```python
from build123d import *

# Parameters (mm, degrees)
SKETCH1_R           = 12.7
BOSS_EXTRUDE1_DEPTH = 622.3
SKETCH2_OUTSIDE_W   = 152.068
SKETCH2_OUTSIDE_H   = 152.068
SKETCH2_OUTSIDE_R   = 6.361935525
CUT_EXTRUDE1_DEPTH  = 38.1
SKETCH5_OUTSIDE_W   = 152.068
SKETCH5_OUTSIDE_H   = 152.068
SKETCH5_OUTSIDE_R   = 6.377907631
CUT_EXTRUDE4_DEPTH  = 38.1


with BuildPart() as part:
    # Sketch1 → Boss-Extrude1 (new body)
    with BuildSketch(Plane.XY):
        Circle(SKETCH1_R)
    extrude(amount=BOSS_EXTRUDE1_DEPTH)

    # Sketch2 outside → Cut-Extrude1 (cut)
    with BuildSketch(Plane.XY):
        Rectangle(SKETCH2_OUTSIDE_W, SKETCH2_OUTSIDE_H)
        with Locations(Location((0, 0, 0), (0, 0, 180))):
            Circle(SKETCH2_OUTSIDE_R, mode=Mode.SUBTRACT)
    extrude(amount=CUT_EXTRUDE1_DEPTH, mode=Mode.SUBTRACT)

    # Sketch5 outside → Cut-Extrude4 (cut)
    with BuildSketch(Plane.XY.offset(622.3)):
        Rectangle(SKETCH5_OUTSIDE_W, SKETCH5_OUTSIDE_H)
        Circle(SKETCH5_OUTSIDE_R, mode=Mode.SUBTRACT)
    extrude(amount=-CUT_EXTRUDE4_DEPTH, mode=Mode.SUBTRACT)


solid = part.part
```
Can you work these out from the model? Positions are in its coordinate system, mm. A direction names the side the tool comes from. Coordinates: 2 decimals unless noted, no trailing zeros. Order: outer loops, then holes, each group sorted by start corner. A loop starts at its lowest first (then second) coordinate and runs counter-clockwise, first axis right, second up. Notation, with made-up numbers: (16.25, 76) - (47.25, 76) arc R25 cw to (47.25, 102) - close; hole circle Ø5 at (26, -25). An arc over 180 degrees is marked (long way). Answer in a Markdown table with one row per item.
1. For pin 1 (1.5 mm diameter, centred on x = -10, z = 71.5, fed in from +Y); pin 2 (2 mm diameter, centred on x = -9, y = -5, fed in from +Z); pin 3 (8 mm diameter, centred on x = 5, z = 352, fed in from +Y), each with a flat end and sliding along its axis, tell me the tip position at first contact or that it passes through.
Reply:
| item | result |
|---|---|
| pin 1 | stops at y = 8.7 |
| pin 2 | stops at z = 584.2 |
| pin 3 | stops at y = 12.66 |
2. For faces 1 (the cylindrical face through (-2.75, -12.4, 307.33)), 2 (the cylindrical face through (6.08, 1.92, 603.52)), 3 (the flat face through (3, 6, 38.1)), which set-ups out of +Z, -Z, +X, -X, +Y, -Y let a thin tool reach every point of the face, with its end or its side?
Reply:
| item | result |
|---|---|
| face 1 | +Z, -Z |
| face 2 | +Z |
| face 3 | -Z |
3. If I drill on line 1 along X through (y, z) = (-1.25, 62); line 2 along Z through (x, y) = (-8.75, 5.5); line 3 along Y through (x, z) = (-0.75, 586), over which ranges is the centre line in solid material (lowest first)?
Reply:
| item | result |
|---|---|
| line 1 | x = -12.64 to 12.64 |
| line 2 | z = 38.1 to 584.2 |
| line 3 | y = -6.33 to 6.33 |
4. Suppose I cut it at A-A (x = 0). Please give me the cut outline in (y, z), and give its area (3 significant figures).
Reply:
| item | result |
|---|---|
| outline | (-12.7, 38.1) - (-6.36, 38.1) - (-6.36, 0) - (6.36, 0) - (6.36, 38.1) - (12.7, 38.1) - (12.7, 584.2) - (6.38, 584.2) - (6.38, 622.3) - (-6.38, 622.3) - (-6.38, 584.2) - (-12.7, 584.2) - close |
| area | 14,800 mm^2 |
5. Suppose I cut it at C-C (z = 577). Please give me the cut outline in (x, y), and give its area (3 significant figures).
Reply:
| item | result |
|---|---|
| outline | circle Ø25.4 at (0, 0) |
| area | 507 mm^2 |
